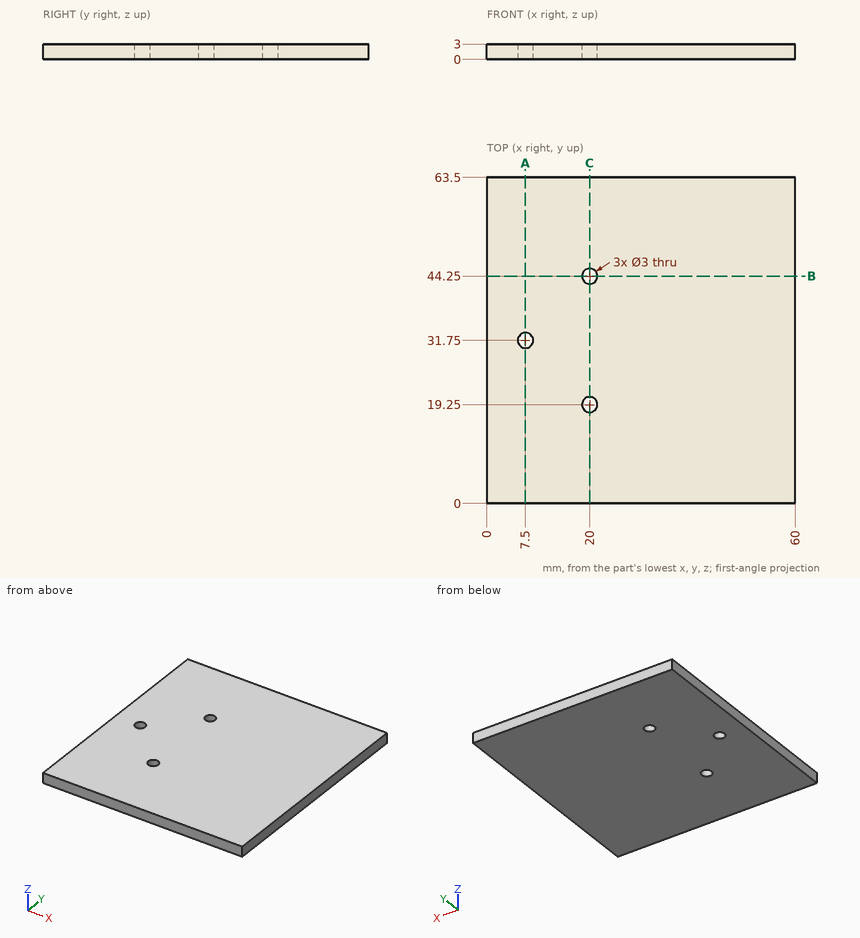
Check sheet for the drawn part. Datum: minimum x, y, z corner. Units: mm. Coordinates: 2 decimals unless noted, no trailing zeros. Write each loop counter-clockwise with the first axis right and the second up, starting at its lowest first coordinate (ties: lowest second). Pieces come first, ordered by that corner, then holes. Notation, with made-up numbers: M 79,43 L 123,43 A24 cw 123,59 Z; hole C 68,-34 d3. An arc over 180 degrees is marked long. Use a Markdown table: item, result.
Q1. Go/stop test with a flat-tipped pin: P1, Ø1.5, axis at x = 53, z = 2, coming from the -Y side. Record where the tip stops, or that it passes through.
Reply:
| item | result |
|---|---|
| P1 | stops at y = 0 |
Q2. Thickness scan on line 1 (Y direction, x = 20, z = 2.35); line 2 (Y direction, x = 7.5, z = 0.95); line 3 (Y direction, x = 6.5, z = 2.9). Record the ranges inside material, lowest first.
Reply:
| item | result |
|---|---|
| line 1 | y = 0 to 17.75, 20.75 to 42.75, 45.75 to 63.5 |
| line 2 | y = 0 to 30.25, 33.25 to 63.5 |
| line 3 | y = 0 to 30.63, 32.87 to 63.5 |
Q3. Sectioned sample at B-B, the plane y = 44.25. Record the boundary of the cut face in (x, z).
Reply:
| item | result |
|---|---|
| outline | M 0,0 L 18.5,0 L 18.5,3 L 0,3 Z; M 21.5,0 L 60,0 L 60,3 L 21.5,3 Z |
Q4. Sectioned sample at C-C, the plane x = 20. Record the boundary of the cut face in (y, z).
Reply:
| item | result |
|---|---|
| outline | M 0,0 L 17.75,0 L 17.75,3 L 0,3 Z; M 20.75,0 L 42.75,0 L 42.75,3 L 20.75,3 Z; M 45.75,0 L 63.5,0 L 63.5,3 L 45.75,3 Z |
Q5. Sectioned sample at A-A, the plane x = 7.5. Record the boundary of the cut face in (y, z), plus the area to 4 significant figures.
Reply:
| item | result |
|---|---|
| outline | M 0,0 L 30.25,0 L 30.25,3 L 0,3 Z; M 33.25,0 L 63.5,0 L 63.5,3 L 33.25,3 Z |
| area | 181.5 mm² |
